Input: part model. Units: mm. Frame: model coordinates. A direction names the side the tool comes from. Give positions to 0.01 mm unless a question says otherwise; leave off trailing zeros. Write each loop counter-clockwise with the first axis right and the second up, starting at its lowest first coordinate (ties: lowest second). Pieces come first, ordered by that corner, then holes. Notation, with made-up numbers: (15, 60.5) - (39, 60.5) arc R11 cw to (39, 80.5) - close; hole circle Ø2 at (67, 42). An arc over 180 degrees is marked (long way). Use a Markdown table: item, result. Add a question column.
1. Pin query (flat end, axial travel): pin 1 (12 mm diameter, centred on y = 89, z = -14.5, fed in from -X); pin 2 (8 mm diameter, centred on y = 196.5, z = 10, fed in from -X); pin 3 (2 mm diameter, centred on x = -14.5, y = 82, fed in from +Z). Return the tip coordinate at first contact, or that it passes through.
2. Section query A-A, the plane y = 187. Return loops of the section in (x, z) (3 decimals).
3. Material intervals for probe 1 along X at (y, z) = (172, 0) (3 decimals); probe 2 along X at (y, z) = (51, -12); probe 3 along Z at (x, y) = (-16, 83.5), sorted ascending.
4. Set-up query: faces 1 (the flat face through (10, 25.4, -30.3)), 2 (the cylindrical face through (30.995, 169.406, 6.883)), 3 (the flat face through (10, 34.036, -30.3)). Return all of +Z, -Z, +X, -X, +Y, -Y with unobstructed straight access to the full face (end or side cutting, diameter ignored); none if empty.
5. Mould query, pull axis Y, two halves, no side actions, for faces 4 (the cylindrical face through (30.995, 84.786, 6.883)), 5 (the cylindrical face through (-10.3, 41.524, -32.707)), 6 (the flat face through (10, 64.77, -30.3)), 7 (the flat face through (10, 97.028, -30.3)). Classes: released by +Y, released by -Y, zero draft, split by the parting line, or undercut.
```python
from build123d import *

# Parameters (mm, degrees)
SKETCH1_R           = 31.75
BOSS_EXTRUDE1_DEPTH = 243.84
SKETCH2_R           = 34.29
BOSS_EXTRUDE2_DEPTH = 0.762
LPATTERN1_COUNT     = 10
LPATTERN1_PITCH     = 7.874
SKETCH3_R           = 29.845
CUT_EXTRUDE1_DEPTH  = 249.61527266


with BuildPart() as part:
    # Sketch1 → Boss-Extrude1 (new body)
    with BuildSketch(Plane(origin=(0, 0, 0), x_dir=(1, 0, 0), z_dir=(0, 1, 0))):
        with Locations(Location((0, 0, 0), (0, 0, 90))):
            Circle(SKETCH1_R)
    extrude(amount=BOSS_EXTRUDE1_DEPTH)

    # Sketch2 → Boss-Extrude2 (add)
    with BuildSketch(Plane(origin=(0, 25.4, 0), x_dir=(1, 0, 0), z_dir=(0, 1, 0))):
        with Locations(Location((0, 0, 0), (0, 0, 90))):
            Circle(SKETCH2_R)
    boss_extrude2 = extrude(amount=BOSS_EXTRUDE2_DEPTH)

    # LPattern1: Boss-Extrude2 ×10
    with Locations(*[(0, i * LPATTERN1_PITCH, 0) for i in range(1, LPATTERN1_COUNT)]):
        add(boss_extrude2)

    # Sketch3 → Cut-Extrude1 (cut, through all)
    with BuildSketch(Plane(origin=(0, 243.84, 0), x_dir=(1, 0, 0), z_dir=(0, 1, 0))):
        with Locations(Location((0, 0, 0), (0, 0, 270))):
            Circle(SKETCH3_R)
    extrude(amount=-CUT_EXTRUDE1_DEPTH, mode=Mode.SUBTRACT)


solid = part.part
```
Result sheet:
| question | item | result |
|---|---|---|
| 1 | pin 1 | stops at x = -33.22 |
| 1 | pin 2 | stops at x = -31.18 |
| 1 | pin 3 | stops at z = 31.39 |
| 2 | outline | circle Ø63.5 at (0, 0); hole circle Ø59.69 at (0, 0) |
| 3 | probe 1 | x = -31.75 to -29.845, 29.845 to 31.75 |
| 3 | probe 2 | x = -29.39 to -27.33, 27.33 to 29.39 |
| 3 | probe 3 | z = -27.42 to -25.19, 25.19 to 27.42 |
| 4 | face 1 | -Y |
| 4 | face 2 | +Y |
| 4 | face 3 | none |
| 5 | face 4 | undercut |
| 5 | face 5 | zero draft |
| 5 | face 6 | undercut |
| 5 | face 7 | released by +Y |
